Verification items for the finished model (mm, model axes). A direction names the side the tool comes from. Give positions to 0.01 mm unless a question says otherwise; leave off trailing zeros. Write each loop counter-clockwise with the first axis right and the second up, starting at its lowest first coordinate (ties: lowest second). Pieces come first, ordered by that corner, then holes. Notation, with made-up numbers: (-20.75, 26.5) -> (36.25, 26.5) arc R28 cw to (36.25, 44.5) -> close; hole circle Ø1 at (4.5, -28). An arc over 180 degrees is marked (long way). Answer as CSV lines item,"result". Start each with the question number.
1) Mould release check, pull along Y, two halves, no side actions. Record for faces 4 (the cylindrical face through (31.291, 23.903, 20.975)), 5 (the flat face through (31, 0, 17)), 6 (the flat face through (31, 22, 0)): released by +Y, released by -Y, zero draft, split by the parting line, or undercut.
2) Sectioned sample at A-A on z = 32.5. Record the cut outline in (x, y).
3) Sectioned sample at B-B on y = 20. Record the cut outline in (x, z), and give its area (3 significant figures).
4) Tool access check on faces 1 (the flat face through (8, 37.817, 17)), 2 (the flat face through (48, 37.817, 17)), 3 (the cylindrical face through (16.37, 44.9, 38.496)). Record the directions out of +Z, -Z, +X, -X, +Y, -Y that give a thin tool (end or side, any length) a straight path to the whole face; none if there is none.
5) Sectioned sample at D-D on x = 50. Record the cut outline in (y, z).
6) Material ranges on L1, parallel to X at y = 52, z = 18; L2, parallel to Y at x = 42.5, z = 3; L3, parallel to Z at x = 56, y = 18.5, recorded low to high.
7) Sectioned sample at C-C on z = 22. Record the cut outline in (x, y).
8) Gauge pin test, flat ends, axial feed: pin 1 Ø1.5 at (x, z) = (35, 32.5) entering from +Y; pin 2 Ø5.5 at (y, z) = (51, 24.5) entering from -X; pin 3 Ø9.5 at (y, z) = (47.5, 16) entering from +X. Record the tip position at first contact, or that the pin passes through.
```python
from build123d import *

# Parameters (mm, degrees)
F0_W     = 16.7905660346
F0_H     = 18.8323240727
F1_DEPTH = 40
F2_R     = 5
F4_D     = 10


with BuildPart() as f1:
    # F0 (on Top) → F1 (new body)
    with BuildSketch(Plane.XY):
        with Locations((23.3397786506, 47.2326790914)):
            Rectangle(F0_W, F0_H)
        Polygon((0, 37.816517055), (0, 0), (63.4701233357, 0), (63.4701233357, 37.816517055), (31.7350616679, 37.816517055), (14.9444956332, 37.816517055), align=None)
    extrude(amount=F1_DEPTH)

    # F2
    f2_edges = [f1.edges().sort_by_distance(p)[0] for p in [
        (31.735062, 47.232679, 40),
        (23.339779, 56.648841, 40),
        (31.735062, 0, 40),
        (0, 18.908259, 40),
        (47.602593, 37.816517, 40),
        (63.470123, 18.908259, 40),
        (14.944496, 47.232679, 40),
        (7.472248, 37.816517, 40),
    ]]
    fillet(f2_edges, radius=F2_R)

    # F4 (through all)
    with Locations(Plane.YZ.offset(63.4701233357)):
        with Locations((18.9082585275, 20.7553303242)):
            Hole(F4_D / 2)


solid = f1.part
```
Ans:
1,face 4,"undercut"
1,face 5,"released by -Y"
1,face 6,"zero draft"
2,outline,"(0, 0) -> (63.47, 0) -> (63.47, 37.82) -> (31.74, 37.82) -> (31.74, 56.65) -> (14.94, 56.65) -> (14.94, 37.82) -> (0, 37.82) -> close"
3,outline,"(0, 0) -> (63.47, 0) -> (63.47, 15.88) -> (0, 15.88) -> close; (0, 25.63) -> (63.47, 25.63) -> (63.47, 35) arc R5 ccw to (58.47, 40) -> (5, 40) arc R5 ccw to (0, 35) -> close"
3,area,"1,910 mm²"
4,face 1,"+Z, -Z, -X, +Y"
4,face 2,"+Z, -Z, +X, +Y"
4,face 3,"+Z, -X, +Y"
5,outline,"(0, 0) -> (37.82, 0) -> (37.82, 35) arc R5 ccw to (32.82, 40) -> (5, 40) arc R5 ccw to (0, 35) -> close; hole circle Ø10 at (18.91, 20.76)"
6,L1,"x = 14.94 to 31.74"
6,L2,"y = 0 to 37.82"
6,L3,"z = 0 to 15.77, 25.74 to 40"
7,outline,"(0, 0) -> (63.47, 0) -> (63.47, 14.07) -> (0, 14.07) -> close; (0, 23.75) -> (63.47, 23.75) -> (63.47, 37.82) -> (31.74, 37.82) -> (31.74, 56.65) -> (14.94, 56.65) -> (14.94, 37.82) -> (0, 37.82) -> close"
8,pin 1,"stops at y = 37.82"
8,pin 2,"stops at x = 14.94"
8,pin 3,"stops at x = 31.74"
